```python
from build123d import *

# Parameters (mm, degrees)
PAD_DEPTH       = 6.5
POCKET_DEPTH    = 6
SKETCH002_R     = 13.5
POCKET001_DEPTH = 1
SKETCH003_W     = 5.4
SKETCH003_H     = 6.5
PAD001_DEPTH    = 3
POCKET002_DEPTH = 10
SKETCH008_R     = 0.6
POCKET003_DEPTH = 2
SKETCH009_R     = 0.6
POCKET004_DEPTH = 2
FILLET_R        = 2.9
FILLET001_R     = 2.9
FILLET002_R     = 5
FILLET003_R     = 5
FILLET004_R     = 5
FILLET005_R     = 5
SKETCH010_W     = 3.95
SKETCH010_H     = 6.5
PAD002_DEPTH    = 3.5
POCKET005_DEPTH = 10
SKETCH012_R     = 0.6
POCKET006_DEPTH = 2
SKETCH013_R     = 0.6
POCKET007_DEPTH = 2
FILLET006_R     = 3.4
FILLET007_R     = 3.4
SKETCH014_R     = 21.6
SKETCH014_R_2   = 20.8
POCKET008_DEPTH = 0.3
SKETCH015_R     = 0.9
PAD003_DEPTH    = 6
FILLET008_R     = 1
POCKET009_DEPTH = 4


with BuildPart() as part:
    # Sketch → Pad (new body)
    with BuildSketch(Plane.XY):
        with BuildLine():
            Line((-22.501992, 16), (-22.501992, -16))
            Line((-22.501992, -16), (-16.285883, -17.9))
            ThreePointArc((-16.285883, -17.9), (0.22069, -24.198994), (16.609636, -17.6))
            Line((16.609636, -17.6), (25.608386, -17.45))
            Line((25.608386, 17.45), (25.608386, -17.45))
            Line((16.609636, 17.6), (25.608386, 17.45))
            ThreePointArc((16.609636, 17.6), (0.22069, 24.198994), (-16.285883, 17.9))
            Line((-22.501992, 16), (-16.285883, 17.9))
        make_face()
    extrude(amount=PAD_DEPTH)

    # Sketch001 → Pocket (cut)
    with BuildSketch(Plane.XY):
        with BuildLine():
            Line((-15.242949, 16.55), (-20.574694, 15.2))
            Line((-20.574694, 15.2), (-20.574694, -15.2))
            Line((-20.574694, -15.2), (-15.242949, -16.55))
            ThreePointArc((-15.242949, -16.55), (0, -22.5), (15.242949, -16.55))
            Line((15.242949, -16.55), (23.527875, -16.05))
            Line((23.527875, 16.05), (23.527875, -16.05))
            Line((15.242949, 16.55), (23.527875, 16.05))
            ThreePointArc((15.242949, 16.55), (0, 22.5), (-15.242949, 16.55))
        make_face()
    extrude(amount=POCKET_DEPTH, mode=Mode.SUBTRACT)

    # Sketch002 (on Face19 of Pocket) → Pocket001 (cut)
    with BuildSketch(Plane(origin=(0, 0, 6), x_dir=(1, 0, 0), z_dir=(0, 0, -1))):
        Circle(SKETCH002_R)
    extrude(amount=-POCKET001_DEPTH, mode=Mode.SUBTRACT)

    # Sketch003 (on Face6 of Pocket001) → Pad001 (join)
    with BuildSketch(Plane.YZ.offset(25.608386)):
        with Locations((-14.75, 3.25)):
            Rectangle(SKETCH003_W, SKETCH003_H)
        with Locations((14.75, 3.25)):
            Rectangle(SKETCH003_W, SKETCH003_H)
    extrude(amount=PAD001_DEPTH)

    # Sketch006 → Pocket002 (cut)
    with BuildSketch(Plane.XY.offset(6.5)):
        with BuildLine():
            ThreePointArc((25.608386, 17.45), (27.01354, 16.442644), (28.608386, 15.775042))
            Line((28.608386, 17.45), (28.608386, 15.775042))
            Line((28.608386, 17.45), (25.608386, 17.45))
        make_face()
        with BuildLine():
            ThreePointArc((28.608386, -15.775042), (27.01354, -16.442644), (25.608386, -17.45))
            Line((28.608386, -17.45), (25.608386, -17.45))
            Line((28.608386, -15.775042), (28.608386, -17.45))
        make_face()
    extrude(amount=-POCKET002_DEPTH, mode=Mode.SUBTRACT)

    # Sketch008 (on Face27 of Pocket002) → Pocket003 (cut)
    with BuildSketch(Plane(origin=(0, -12.05, 0), x_dir=(-1, 0, 0), z_dir=(0, 1, 0))):
        with Locations((-26.908386, 1.7)):
            Circle(SKETCH008_R)
    extrude(amount=-POCKET003_DEPTH, mode=Mode.SUBTRACT)

    # Sketch009 (on Face26 of Pocket003) → Pocket004 (cut)
    with BuildSketch(Plane.XZ.offset(-12.05)):
        with Locations((26.908386, 1.7)):
            Circle(SKETCH009_R)
    extrude(amount=-POCKET004_DEPTH, mode=Mode.SUBTRACT)

    # Fillet
    fillet_edges = [part.edges().sort_by_distance(p)[0] for p in [
        (28.608386, -13.912521, 6.5),
    ]]
    fillet(fillet_edges, radius=FILLET_R)

    # Fillet001
    fillet001_edges = [part.edges().sort_by_distance(p)[0] for p in [
        (28.608386, 13.912521, 6.5),
    ]]
    fillet(fillet001_edges, radius=FILLET001_R)

    # Fillet002
    fillet002_edges = [part.edges().sort_by_distance(p)[0] for p in [
        (16.609636, -17.6, 3.25),
    ]]
    fillet(fillet002_edges, radius=FILLET002_R)

    # Fillet003
    fillet003_edges = [part.edges().sort_by_distance(p)[0] for p in [
        (16.609636, 17.6, 3.25),
    ]]
    fillet(fillet003_edges, radius=FILLET003_R)

    # Fillet004
    fillet004_edges = [part.edges().sort_by_distance(p)[0] for p in [
        (-16.285883, -17.9, 3.25),
    ]]
    fillet(fillet004_edges, radius=FILLET004_R)

    # Fillet005
    fillet005_edges = [part.edges().sort_by_distance(p)[0] for p in [
        (-16.285883, 17.9, 3.25),
    ]]
    fillet(fillet005_edges, radius=FILLET005_R)

    # Sketch010 (on Face4 of Fillet005) → Pad002 (join)
    with BuildSketch(Plane(origin=(-22.501992, 0, 0), x_dir=(0, -1, 0), z_dir=(-1, 0, 0))):
        with Locations((-14.025, 3.25)):
            Rectangle(SKETCH010_W, SKETCH010_H)
        with Locations((14.025, 3.25)):
            Rectangle(SKETCH010_W, SKETCH010_H)
    extrude(amount=PAD002_DEPTH)

    # Sketch011 (on Face6 of Pad002) → Pocket005 (cut)
    with BuildSketch(Plane.XY.offset(6.5)):
        with BuildLine():
            ThreePointArc((-26.001992, 14.6), (-24.192608, 15.15154), (-22.501992, 16))
            Line((-22.501992, 16), (-26.001992, 16))
            Line((-26.001992, 16), (-26.001992, 14.6))
        make_face()
        with BuildLine():
            ThreePointArc((-22.501992, -16), (-24.192608, -15.15154), (-26.001992, -14.6))
            Line((-26.001992, -14.6), (-26.001992, -16))
            Line((-26.001992, -16), (-22.501992, -16))
        make_face()
    extrude(amount=-POCKET005_DEPTH, mode=Mode.SUBTRACT)

    # Sketch012 (on Face23 of Pocket005) → Pocket006 (cut)
    with BuildSketch(Plane(origin=(0, -12.05, 0), x_dir=(-1, 0, 0), z_dir=(0, 1, 0))):
        with Locations((24.301992, 1.7)):
            Circle(SKETCH012_R)
    extrude(amount=-POCKET006_DEPTH, mode=Mode.SUBTRACT)

    # Sketch013 (on Face21 of Pocket006) → Pocket007 (cut)
    with BuildSketch(Plane.XZ.offset(-12.05)):
        with Locations((-24.301992, 1.7)):
            Circle(SKETCH013_R)
    extrude(amount=-POCKET007_DEPTH, mode=Mode.SUBTRACT)

    # Fillet006
    fillet006_edges = [part.edges().sort_by_distance(p)[0] for p in [
        (-26.001992, 13.325, 6.5),
    ]]
    fillet(fillet006_edges, radius=FILLET006_R)

    # Fillet007
    fillet007_edges = [part.edges().sort_by_distance(p)[0] for p in [
        (-26.001992, -13.325, 6.5),
    ]]
    fillet(fillet007_edges, radius=FILLET007_R)

    # Sketch014 (on Face4 of Fillet007) → Pocket008 (cut)
    with BuildSketch(Plane.XY.offset(6.5)):
        Circle(SKETCH014_R)
        Circle(SKETCH014_R_2, mode=Mode.SUBTRACT)
    extrude(amount=-POCKET008_DEPTH, mode=Mode.SUBTRACT)

    # Sketch015 (on Face55 of Pocket008) → Pad003 (join)
    with BuildSketch(Plane(origin=(0, 0, 6), x_dir=(1, 0, 0), z_dir=(0, 0, -1))):
        with Locations((-18.42, 13.32)):
            Circle(SKETCH015_R)
        with Locations((-18.42, -13.32)):
            Circle(SKETCH015_R)
        with Locations((7.27, 18.56)):
            Circle(SKETCH015_R)
        with Locations((5.37, -19.79)):
            Circle(SKETCH015_R)
    extrude(amount=PAD003_DEPTH)

    # Fillet008
    fillet008_edges = [part.edges().sort_by_distance(p)[0] for p in [
        (-19.32, -13.32, 6),
        (6.37, -18.56, 6),
        (-19.32, 13.32, 6),
        (4.47, 19.79, 6),
    ]]
    fillet(fillet008_edges, radius=FILLET008_R)

    # Sketch016 (on Face16 of Fillet008) → Pocket009 (cut)
    with BuildSketch(Plane(origin=(0, 0, 0), x_dir=(1, 0, 0), z_dir=(0, 0, -1))):
        with BuildLine():
            Line((-5, 23.677838), (-5, 21.937411))
            ThreePointArc((5, 21.937411), (0, 22.5), (-5, 21.937411))
            Line((5, 23.677838), (5, 21.937411))
            ThreePointArc((5, 23.677838), (0, 24.2), (-5, 23.677838))
        make_face()
    extrude(amount=-POCKET009_DEPTH, mode=Mode.SUBTRACT)


solid = part.part
```
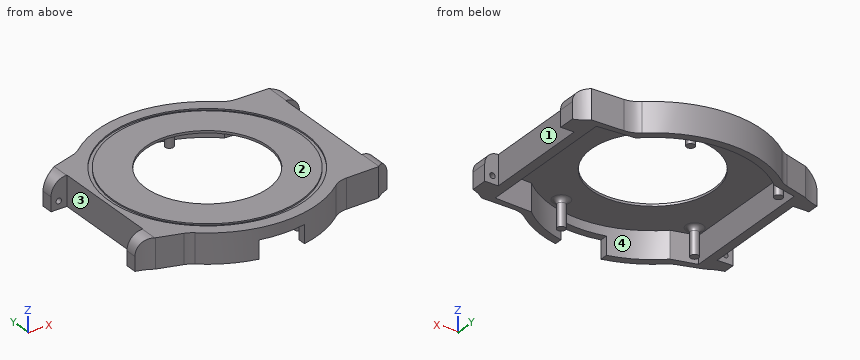
Verification items for the finished model (mm, model axes). Face numbers are marked on the shaded views. A direction names the side the tool comes from. Coordinates: 2 decimals unless noted, no trailing zeros. Loops run counter-clockwise (first coordinate to the right, second up) from the corner with the lowest first, then second, coordinate; pieces in that order, holes last. Notation, with made-up numbers: (-35, -26.5) -> (15, -26.5) arc R16 cw to (15, -1.5) -> close; hole circle Ø8 at (45.5, 48). An arc over 180 degrees is marked (long way). Answer in a Markdown table with one row per item. Add a question column.
1. Section check D-D, the plane y = 19.79. Enter the section's corners in (x, z), then the cut area to 3 significant figures.
2. Access from +Z, -Z, +X, -X, +Y, -Y to the whole of each face (thin tool, end or side, straight path). Record for the marked faces 1, 2, 3 and 4.
3. Section check C-C, the plane x = 14.5. Enter the section's corners in (y, z).
4. Section check A-A, the plane x = 0. Enter the section's corners in (y, z).
5. Section check B-B, the plane y = 3. Enter the section's corners in (x, z).
6. Material ranges on probe 1 along Y at (x, z) = (0, 6.3); probe 2 along X at (y, z) = (-4, 0.5); probe 3 along Z at (x, y) = (-12.5, -13), recorded low to high. Write a range as [from, to].
7. Depth check by flat-ended pin: P1, Ø1, axis at x = 13.5, y = -14.5, coming from the -Z side; P2, Ø0.7, axis at x = 26.91, z = 1.7, coming from the -Y side; P3, Ø0.9, axis at x = 26.5, z = 4.5, coming from the -Y side. Enter the tip coordinate at first touch or a pass-through.
Derived:
| question | item | result |
|---|---|---|
| 1 | outline | (-13.93, 0) -> (-10.71, 0) -> (-10.71, 6) -> (3.47, 6) arc R1 cw to (4.47, 5) -> (4.47, 0) -> (6.27, 0) -> (6.27, 5) arc R1 cw to (7.27, 6) -> (10.71, 6) -> (10.71, 0) -> (13.93, 0) -> (13.93, 6.5) -> (8.66, 6.5) -> (8.66, 6.2) -> (6.4, 6.2) -> (6.4, 6.5) -> (-6.4, 6.5) -> (-6.4, 6.2) -> (-8.66, 6.2) -> (-8.66, 6.5) -> (-13.93, 6.5) -> close |
| 1 | area | 62.5 mm² |
| 2 | face 1 | +Z, -Z, +X |
| 2 | face 2 | +Z, +X, -X, +Y, -Y |
| 2 | face 3 | +Z, -Z, -X |
| 2 | face 4 | -Z |
| 3 | outline | (-19.37, 0) -> (-17.2, 0) -> (-17.2, 6) -> (17.2, 6) -> (17.2, 0) -> (19.37, 0) -> (19.37, 6.5) -> (16.01, 6.5) -> (16.01, 6.2) -> (14.91, 6.2) -> (14.91, 6.5) -> (-14.91, 6.5) -> (-14.91, 6.2) -> (-16.01, 6.2) -> (-16.01, 6.5) -> (-19.37, 6.5) -> close |
| 4 | outline | (-24.2, 4) -> (-22.5, 4) -> (-22.5, 6) -> (-13.5, 6) -> (-13.5, 6.5) -> (-20.8, 6.5) -> (-20.8, 6.2) -> (-21.6, 6.2) -> (-21.6, 6.5) -> (-24.2, 6.5) -> close; (13.5, 6) -> (22.5, 6) -> (22.5, 0) -> (24.2, 0) -> (24.2, 6.5) -> (21.6, 6.5) -> (21.6, 6.2) -> (20.8, 6.2) -> (20.8, 6.5) -> (13.5, 6.5) -> close |
| 5 | outline | (-22.5, 0) -> (-20.57, 0) -> (-20.57, 6) -> (-13.16, 6) -> (-13.16, 6.5) -> (-20.58, 6.5) -> (-20.58, 6.2) -> (-21.39, 6.2) -> (-21.39, 6.5) -> (-22.5, 6.5) -> close; (13.16, 6) -> (23.53, 6) -> (23.53, 0) -> (25.61, 0) -> (25.61, 6.5) -> (21.39, 6.5) -> (21.39, 6.2) -> (20.58, 6.2) -> (20.58, 6.5) -> (13.16, 6.5) -> close |
| 6 | probe 1 | y = [-24.2, -21.6], [-20.8, -13.5], [13.5, 20.8], [21.6, 24.2] |
| 6 | probe 2 | x = [-22.5, -20.57], [23.53, 25.61] |
| 6 | probe 3 | z = [6, 6.5] |
| 7 | P1 | stops at z = 6 |
| 7 | P2 | stops at y = -16.72 |
| 7 | P3 | stops at y = -17.08 |
